Read the model definition and answer for the solid it produces. Units are mm, in the model's axes. A direction names the side the tool comes from. Give positions to 0.01 mm unless a question says otherwise; leave off trailing zeros. Order: outer loops, then holes, each group sorted by start corner. A loop starts at its lowest first (then second) coordinate and runs counter-clockwise, first axis right, second up. Notation, with made-up numbers: (-23, 51.5) -> (12, 51.5) arc R30 cw to (12, 86.5) -> close; hole circle Ø1 at (-31.75, 56). An arc over 180 degrees is marked (long way). Use one line per item in the form item = value.
```python
from build123d import *

# Parameters (mm, degrees)
SKETCH1_W               = 64
SKETCH1_H               = 38
BOSS_EXTRUDE1_DEPTH     = 16
CUT_EXTRUDE2_START      = 10
SKETCH3_R               = 11.5
CUT_EXTRUDE2_DEPTH      = 10
CUT_EXTRUDE3_DEPTH      = 41.509258201
CUT_EXTRUDE3_DEPTH_BACK = 41.509258201
SKETCH5_R               = 2
BATTERY_DEPTH           = 22
BATTERY_DEPTH_BACK      = 14
SKETCH4_R               = 9
CUT_EXTRUDE4_REACH      = 45.509
CUT_EXTRUDE4_START      = 3
SKETCH6_W               = 17
SKETCH6_H               = 5
SKETCH7_W               = 12
SKETCH7_H               = 8
CUT_EXTRUDE5_DEPTH      = 3
FILLET1_R               = 1.5
SKETCH8_R               = 5.5
CUT_EXTRUDE6_DEPTH      = 10


with BuildPart() as part:
    # Sketch1 → Boss-Extrude1 (new body)
    with BuildSketch(Plane(origin=(0, 0, 0), x_dir=(1, 0, 0), z_dir=(0, 1, 0))):
        Rectangle(SKETCH1_W, SKETCH1_H)
    extrude(amount=BOSS_EXTRUDE1_DEPTH)

    # Sketch3 → Cut-Extrude2 (cut)
    with BuildSketch(Plane.XY.offset(CUT_EXTRUDE2_START)):
        with BuildLine():
            Line((36.5, -6.5), (36.5, 5))
            ThreePointArc((36.5, 5), (33.131727984, -3.131727984), (25, -6.5))
            Line((25, -6.5), (36.5, -6.5))
        make_face()
        with Locations((25, 5)):
            Circle(SKETCH3_R)
        with BuildLine():
            Line((36.5, 16.5), (25, 16.5))
            ThreePointArc((25, 16.5), (33.131727984, 13.131727984), (36.5, 5))
            Line((36.5, 5), (36.5, 16.5))
        make_face()
        with Locations((-25, 5)):
            Circle(SKETCH3_R)
        with BuildLine():
            Line((-36.5, -6.5), (-25, -6.5))
            ThreePointArc((-25, -6.5), (-33.131727957, -3.13172801), (-36.5, 4.999999925))
            Line((-36.5, 4.999999925), (-36.5, -6.5))
        make_face()
        with BuildLine():
            Line((-36.5, 16.5), (-36.5, 4.999999925))
            ThreePointArc((-36.5, 4.999999925), (-33.13172801, 13.131727957), (-25, 16.5))
            Line((-25, 16.5), (-36.5, 16.5))
        make_face()
    cut_extrude2 = extrude(amount=CUT_EXTRUDE2_DEPTH, mode=Mode.SUBTRACT)

    # Mirror1: Cut-Extrude2 across plane
    add(cut_extrude2.mirror(Plane.XY), mode=Mode.SUBTRACT)

    # Sketch5 → Cut-Extrude3 (cut, two sides: drawn at the far end of the back side and taken through both)
    with BuildSketch(Plane.XY.offset(-CUT_EXTRUDE3_DEPTH_BACK)):
        with Locations((25, 5)):
            Circle(SKETCH5_R)
        with Locations((-25, 5)):
            Circle(SKETCH5_R)
    extrude(amount=CUT_EXTRUDE3_DEPTH + CUT_EXTRUDE3_DEPTH_BACK, mode=Mode.SUBTRACT)


with BuildPart() as body_2:
    # Sketch4 → Battery (new, two sides: drawn at the far end of the back side and taken through both)
    with BuildSketch(Plane(origin=(0, 0, 0), x_dir=(0, 0, -1), z_dir=(1, 0, 0)).offset(-BATTERY_DEPTH_BACK)):
        with Locations((0, 12)):
            Circle(SKETCH4_R)
        with BuildLine():
            Line((-9, 23.052760149), (-9, 12))
            ThreePointArc((-9, 12), (0, 21), (9, 12))
            Line((9, 12), (9, 23.052760149))
            Line((9, 23.052760149), (-9, 23.052760149))
        make_face()
    extrude(amount=BATTERY_DEPTH + BATTERY_DEPTH_BACK)


with BuildPart() as part_1:
    add(part.part)

    # Combine1: cut body 2
    add(body_2.part, mode=Mode.SUBTRACT)

    # Sketch6 → Cut-Extrude4 (cut, up to next)
    with BuildSketch(Plane(origin=(0, 0, 0), x_dir=(1, 0, 0), z_dir=(0, 1, 0)).offset(CUT_EXTRUDE4_START), mode=Mode.PRIVATE) as cut_extrude4_sk1:
        with Locations((0, 13)):
            Rectangle(SKETCH6_W, SKETCH6_H)
    cut_extrude4_tool1 = extrude(cut_extrude4_sk1.sketch, amount=CUT_EXTRUDE4_REACH, mode=Mode.PRIVATE) & part_1.part
    add(cut_extrude4_tool1.solids().sort_by_distance((0, 3, -13))[0], mode=Mode.SUBTRACT)

    # Sketch7 → Cut-Extrude5 (cut)
    with BuildSketch(Plane.XZ):
        with Locations((0, -13)):
            Rectangle(SKETCH7_W, SKETCH7_H)
    extrude(amount=-CUT_EXTRUDE5_DEPTH, mode=Mode.SUBTRACT)

    # Fillet1
    fillet1_edges = [part_1.edges().sort_by_distance(p)[0] for p in [
        (0, 3, -17),
        (0, 3, -9),
    ]]
    fillet(fillet1_edges, radius=FILLET1_R - 0.0001)  # a hair under: the kernel refuses the full size

    # Sketch8 → Cut-Extrude6 (cut, symmetric)
    with BuildSketch(Plane.XY):
        with Locations((-20, 15)):
            Circle(SKETCH8_R)
    extrude(amount=CUT_EXTRUDE6_DEPTH, both=True, mode=Mode.SUBTRACT)


solid = part_1.part
```
Item 1: The part is cut by section D-D on z = 0. Give the vertices of the cut face in (x, y).
Checks:
outline = (-32, 0) -> (32, 0) -> (32, 16) -> (22, 16) -> (22, 3) -> (-14, 3) -> (-14, 16) -> (-14.59, 16) arc R5.5 cw (long way) to (-25.41, 16) -> (-32, 16) -> close; hole circle Ø4 at (-25, 5); hole circle Ø4 at (25, 5)
Item 2: Which of the six approach directions +Z, -Z, +X, -X, +Y, -Y give full straight-line access (tool end or side, diameter ignored) to faces 1 (the cylindrical face through (-20.1, 9.5, 0.1)), 2 (the flat face through (4, 14, -9)), 3 (the flat face through (6, 1, -13)), 4 (the cylindrical face through (14.521, 9.737, -14.437))?
Checks:
face_1 = none
face_2 = +Y
face_3 = -Y
face_4 = -Z, +X
Item 3: The part is cut by section A-A on y = 5. Give the vertices of the cut face in (x, z).
Checks:
outline = (-32, -10) -> (-27, -10) -> (-27, 10) -> (-32, 10) -> close; (-23, -10) -> (-13.5, -10) -> (-13.5, -19) -> (13.5, -19) -> (13.5, -10) -> (23, -10) -> (23, 10) -> (13.5, 10) -> (13.5, 19) -> (-13.5, 19) -> (-13.5, 10) -> (-23, 10) -> close; (27, -10) -> (32, -10) -> (32, 10) -> (27, 10) -> close; hole (-14, -5.66) -> (22, -5.66) -> (22, 5.66) -> (-14, 5.66) -> close; hole (-8.5, -15.5) -> (8.5, -15.5) -> (8.5, -10.5) -> (-8.5, -10.5) -> close
Item 4: Determine the mould class of faces 5 (the flat face through (0, 9, -15.5)), 6 (the cylindrical face through (14.521, 9.737, 14.437)), 7 (the flat face through (-29, 16, 0)) for opening direction X: +X half, -X half, draft (parallel to the pull), parting line (faces both ways), or undercut.
Checks:
face_5 = undercut
face_6 = +X half
face_7 = draft
Item 5: Straight lines are drawn through the part: L1, parallel to X at y = 5, z = 3.25; L2, parallel to Z at x = 4.5, y = 15.75; L3, parallel to X at y = 15, z = -0.5. For each, find the intervals that lie inside material, in ascending order. Write a range as from..to.
Checks:
L1 = -32..-27, -23..-14, 22..23, 27..32
L2 = -19..-15.5, -10.5..-9, 9..19
L3 = -32..-25.5, -14.5..-14, 22..32
Item 6: Given pin 1 Ø8 at (x, y) = (-20.5, 8.5) entering from +Z; pin 2 Ø8 at (x, y) = (-22, 4.5) entering from -Z; pin 3 Ø2.5 at (x, y) = (-25, 5) entering from -Z; pin 4 Ø2.5 at (y, z) = (1, -12.5) entering from +X, each flat-ended and moving along its own axis, determine where each tip first touches the part or whether it passes through.
Checks:
pin_1 = 10
pin_2 = -10
pin_3 = through
pin_4 = 14.64
Item 7: The part is cut by section C-C on y = 15. Give the vertices of the cut face in (x, z).
Checks:
outline = (-32, -10) -> (-25.5, -10) -> (-25.5, 10) -> (-32, 10) -> close; (-19.32, -19) -> (19.32, -19) -> (19.32, -10) -> (32, -10) -> (32, 10) -> (19.32, 10) -> (19.32, 19) -> (-19.32, 19) -> (-19.32, 10) -> (-14.5, 10) -> (-14.5, -10) -> (-19.32, -10) -> close; hole (-14, -9) -> (22, -9) -> (22, 9) -> (-14, 9) -> close; hole (-8.5, -15.5) -> (8.5, -15.5) -> (8.5, -10.5) -> (-8.5, -10.5) -> close
